Here's how the part is built. I have some questions about the finished solid (model axes, mm). A direction names the side the tool comes from. Give positions to 0.01 mm unless a question says otherwise; leave off trailing zeros. Order: outer loops, then holes, each group sorted by start corner. A loop starts at its lowest first (then second) coordinate and runs counter-clockwise, first axis right, second up. Notation, with made-up numbers: M 47,57 L 67,57 A5 cw 67,65 Z; hole C 82,-6.5 d11. An arc over 180 degrees is marked long. Use one line per item in the form item = value.
from build123d import *

# Parameters (mm, degrees)
SKETCH1_W           = 50.8
SKETCH1_H           = 198.12
SKETCH1_R           = 1.1303
SKETCH1_R_2         = 7.62
BOSS_EXTRUDE1_DEPTH = 6.35
SKETCH2_R           = 5.08
CUT_EXTRUDE1_DEPTH  = 6.35
CHAMFER1_SIZE       = 12.54
CHAMFER1_SIZE2      = 143.332855877
FILLET1_R           = 10
CUT_EXTRUDE2_DEPTH  = 10.668


with BuildPart() as part:
    # Sketch1 → Boss-Extrude1 (new body)
    with BuildSketch(Plane(origin=(0, 0, 0), x_dir=(1, 0, 0), z_dir=(0, 1, 0))):
        with Locations((25.4, 99.06)):
            Rectangle(SKETCH1_W, SKETCH1_H)
        with Locations(Location((12.7, 19.05, 0), (0, 0, 270))):
            Circle(SKETCH1_R, mode=Mode.SUBTRACT)
        with Locations(Location((38.1, 19.05, 0), (0, 0, 270))):
            Circle(SKETCH1_R, mode=Mode.SUBTRACT)
        with Locations(Location((25.4, 19.05, 0), (0, 0, 270))):
            Circle(SKETCH1_R_2, mode=Mode.SUBTRACT)
    extrude(amount=BOSS_EXTRUDE1_DEPTH)

    # Sketch2 → Cut-Extrude1 (cut)
    with BuildSketch(Plane(origin=(0, 6.35, 0), x_dir=(1, 0, 0), z_dir=(0, 1, 0))):
        with Locations(Location((25.4, 172.72, 0), (0, 0, 270))):
            Circle(SKETCH2_R)
        with Locations(Location((25.4, 147.32, 0), (0, 0, 270))):
            Circle(SKETCH2_R)
    extrude(amount=-CUT_EXTRUDE1_DEPTH, mode=Mode.SUBTRACT)

    # Chamfer1
    chamfer1_edges = [part.edges().sort_by_distance(p)[0] for p in [
        (0, 3.175, -198.12),
        (50.8, 3.175, -198.12),
    ]]
    chamfer1_side = [part.faces().sort_by_distance(p)[0] for p in [
        (25.4, 3.175, -198.12),
    ]]
    chamfer(chamfer1_edges, length=CHAMFER1_SIZE, length2=CHAMFER1_SIZE2, reference=chamfer1_side[0])

    # Fillet1
    fillet1_edges = [part.edges().sort_by_distance(p)[0] for p in [
        (12.54, 3.175, -198.12),
        (38.26, 3.175, -198.12),
    ]]
    fillet(fillet1_edges, radius=FILLET1_R)

    # Sketch3 → Cut-Extrude2 (cut)
    with BuildSketch(Plane(origin=(0, 6.35, 0), x_dir=(1, 0, 0), z_dir=(0, 1, 0))):
        with BuildLine():
            Line((9.459358265, 77.6224), (41.340641735, 77.6224))
            ThreePointArc((41.340641735, 77.6224), (42.763041735, 76.2), (41.340641735, 74.7776))
            Line((41.340641735, 74.7776), (9.459358265, 74.7776))
            ThreePointArc((9.459358265, 74.7776), (8.036958265, 76.2), (9.459358265, 77.6224))
        make_face()
    extrude(amount=-CUT_EXTRUDE2_DEPTH, mode=Mode.SUBTRACT)


solid = part.part
Q1. I want a section at B-B on x = 25.4. Write out the boundary of the cut face in (y, z).
Found:
outline = M 0,-198.12 L 6.35,-198.12 L 6.35,-177.8 L 0,-177.8 Z; M 0,-167.64 L 6.35,-167.64 L 6.35,-152.4 L 0,-152.4 Z; M 0,-142.24 L 6.35,-142.24 L 6.35,-77.62 L 0,-77.62 Z; M 0,-74.78 L 6.35,-74.78 L 6.35,-26.67 L 0,-26.67 Z; M 0,-11.43 L 6.35,-11.43 L 6.35,0 L 0,0 Z
Q2. I need wall thicknesses on L1, parallel to X at y = 2.5, z = -19.05; L2, parallel to Z at x = 25, y = 1.5; L3, parallel to Z at x = 21.5, y = 6.25. Which ranges of each line are inside material? Lowest first, please.
Found:
L1 = 0 to 11.57, 13.83 to 17.78, 33.02 to 36.97, 39.23 to 50.8
L2 = -198.12 to -177.78, -167.66 to -152.38, -142.26 to -77.62, -74.78 to -26.66, -11.44 to 0
L3 = -198.12 to -175.98, -169.46 to -150.58, -144.06 to -77.62, -74.78 to -25.6, -12.5 to 0
Q3. I'm going to push flat-ended pins straight in: pin 1 Ø24.5 at (x, z) = (25.4, -19.05) entering from +Y; pin 2 Ø8 at (x, z) = (25.4, -172.72) entering from -Y; pin 3 Ø2 at (x, y) = (16.5, 3.5) entering from -Z; pin 4 Ø2 at (y, z) = (1, -60) entering from -X. Where does each tip first touch, or does it pass through?
Found:
pin_1 = 6.35
pin_2 = through
pin_3 = -197.19
pin_4 = 0.37
Q4. I want a section at D-D on z = -172.72. Write out the boundary of the cut face in (x, y), then the cut area to 3 significant figures.
Found:
outline = M 10.32,0 L 20.32,0 L 20.32,6.35 L 10.32,6.35 Z; M 30.48,0 L 40.48,0 L 40.48,6.35 L 30.48,6.35 Z
area = 127 mm²
Q5. Thinking about a two-plate mould opening in Z: for faces 1 (the face through (25, 3, -198.12)), 2 (the face through (0, 3, -27)), 3 (the face through (26, 3, -74.778)), 4 (the face through (26.926, 3.219, -167.875)), which applies, +Z half, -Z half, draft (parallel to the pull), parting line (faces both ways), or undercut?
Found:
face_1 = -Z half
face_2 = draft
face_3 = undercut
face_4 = undercut
Q6. I want a section at A-A on y = 4.5. Write out the boundary of the cut face in (x, z).
Found:
outline = M 0,-54.79 L 11.74,-188.99 A10 ccw 21.7,-198.12 L 29.1,-198.12 A10 ccw 39.06,-188.99 L 50.8,-54.79 L 50.8,0 L 0,0 Z; hole M 9.46,-77.62 L 41.34,-77.62 A1.42 ccw 41.34,-74.78 L 9.46,-74.78 A1.42 ccw Z; hole C 12.7,-19.05 d2.26; hole C 25.4,-19.05 d15.24; hole C 25.4,-172.72 d10.16; hole C 25.4,-147.32 d10.16; hole C 38.1,-19.05 d2.26
Q7. On a 3-axis mill with a long thin cutter (end or side, diameter ignored), from which of +Z, -Z, +X, -X, +Y, -Y can I reach the whole of each face in a straight line? I mean faces 5 (the face through (35.78, 3.22, -195.56)), 6 (the face through (25, 3, -77.622)). Say none if no direction works.
Found:
face_5 = -Z, +X, +Y, -Y
face_6 = +Y, -Y
Q8. I want a section at C-C on z = -147.32. Write out the boundary of the cut face in (x, y).
Found:
outline = M 8.1,0 L 20.32,0 L 20.32,6.35 L 8.1,6.35 Z; M 30.48,0 L 42.7,0 L 42.7,6.35 L 30.48,6.35 Z
